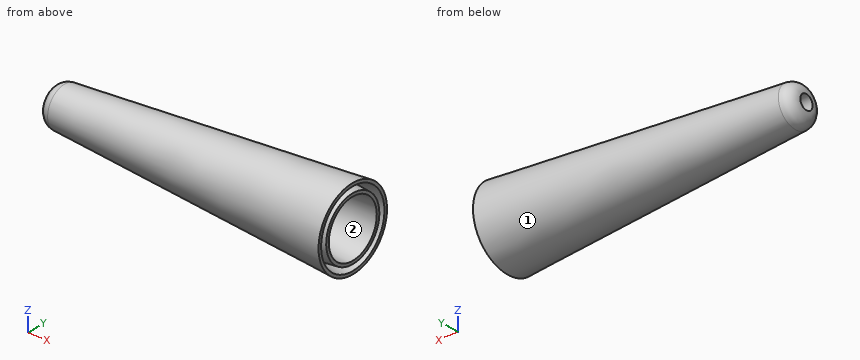
```python
from build123d import *


with BuildPart() as part:
    # Sketch2 → Revolve2 (revolve)
    with BuildSketch(Plane.XY, mode=Mode.PRIVATE) as revolve2_sk:
        with BuildLine():
            Line((0, 1.2), (50, 4.696340597))
            Line((50, 4.696340597), (50, 6.696340597))
            Line((50, 6.696340597), (1.851094968, 3.32944117))
            ThreePointArc((1.851094968, 3.32944117), (0.484525778, 2.648094905), (0, 1.2))
        make_face()
    revolve(revolve2_sk.sketch.rotate(Axis((-19.275847123, 0, 0), (1, 0, 0)), 90), axis=Axis((-19.275847123, 0, 0), (1, 0, 0)))

    # Sketch3 → Revolve3 (revolve)
    with BuildSketch(Plane.XY, mode=Mode.PRIVATE) as revolve3_sk:
        Polygon((50, 4.695121509), (180, 9.234821543), (180, 11.236040631), (50, 6.696340597), align=None)
    revolve(revolve3_sk.sketch.rotate(Axis((50, 0, 0), (-1, 0, 0)), 90), axis=Axis((50, 0, 0), (-1, 0, 0)))

    # SurfaceCut3
    split(bisect_by=Plane(origin=(50, 0, 0), x_dir=(0, 0, -1), z_dir=(1, 0, 0)), keep=Keep.BOTTOM)

    # Sketch4 → Cut-Revolve1 (revolve, cut)
    with BuildSketch(Plane.XY, mode=Mode.PRIVATE) as cut_revolve1_sk:
        Polygon((50, 6.195119648), (47, 5.484118263), (50, 5.196340597), align=None)
    revolve(cut_revolve1_sk.sketch.rotate(Axis((50, 0, 0), (-1, 0, 0)), 90), axis=Axis((50, 0, 0), (-1, 0, 0)), mode=Mode.SUBTRACT)


solid = part.part
```
CAD build for the part. Positions are in the model's coordinates, mm. Face numbers are marked on the shaded views. Coordinates: 2 decimals unless noted, no trailing zeros. Order: outer loops, then holes, each group sorted by start corner. A loop starts at its lowest first (then second) coordinate and runs counter-clockwise, first axis right, second up.
(1) Mould opens along Z. For the marked faces 1 and 2 say: released by +Z, released by -Z, zero draft, split by the parting line, or undercut.
Solution:
face 1: split by the parting line
face 2: undercut
(2) Saw through at B-B, the plane x = 16. Write the cut outline in (y, z).
Solution:
outline: circle Ø8.64 at (0, 0); hole circle Ø4.64 at (0, 0)
(3) Saw through at A-A, the plane x = 46. Write the cut outline in (y, z), and give its area (3 significant figures).
Solution:
outline: circle Ø12.83 at (0, 0); hole circle Ø8.83 at (0, 0)
area: 68.1 mm2
(4) Pin check, flat tips, straight feed: pin 1 Ø5 at (x, y) = (37.5, -2) entering from +Z; pin 2 Ø8 at (x, y) = (28, -3.5) entering from +Z; pin 3 Ø1.5 at (x, z) = (12, 0.5) entering from +Y; pin 4 Ø1.5 at (y, z) = (-5, 3.5) entering from +X. Stop position of each tip, or through.
Solution:
pin 1: stops at z = 5.94
pin 2: stops at z = 5.32
pin 3: stops at y = 4.08
pin 4: stops at x = 50
(5) Drill centre lines: L1, parallel to Z at x = 31, y = -0.25; L2, parallel to Z at x = 23.5, y = 1.5; L3, parallel to Y at x = 24.5, z = -0.75 (3 decimals). Where is each one in solid material? Low to high.
Solution:
L1: z = -5.36 to -3.36, 3.36 to 5.36
L2: z = -4.61 to -2.42, 2.42 to 4.61
L3: y = -4.856 to -2.815, 2.815 to 4.856
